The model under review builds one solid part; all positions refer to its coordinate system, in mm. A direction names the side the tool comes from. Give positions to 0.01 mm unless a question says otherwise; leave off trailing zeros. Order: outer loops, then holes, each group sorted by start corner. A loop starts at its lowest first (then second) coordinate and runs counter-clockwise, first axis right, second up. Notation, with made-up numbers: (48, 38) - (101, 38) arc R35 cw to (101, 72) - close; hole circle Ø10 at (35, -25.5). An arc over 180 degrees is marked (long way). Use CSV: the item, a comma, the result in double quotes. Start each with the question number.
```python
from build123d import *

# Parameters (mm, degrees)
F0_W     = 215.9
F0_H     = 50.8
F0_R     = 2.5527
F0_R_2   = 14.2875
F1_DEPTH = 25.4
F2_W     = 22.225
F2_H     = 47.625
F3_DEPTH = 215.901
F4_R     = 2.5527
F5_DEPTH = 50.801


with BuildPart() as f1:
    # F0 (on Front) → F1 (new body)
    with BuildSketch(Plane.XZ):
        Rectangle(F0_W, F0_H)
        with Locations((-57.15, -12.7)):
            Circle(F0_R, mode=Mode.SUBTRACT)
        with Locations((-31.75, -12.7)):
            Circle(F0_R, mode=Mode.SUBTRACT)
        with Locations((-6.35, -12.7)):
            Circle(F0_R, mode=Mode.SUBTRACT)
        with Locations((-82.55, 0)):
            Circle(F0_R_2, mode=Mode.SUBTRACT)
        with Locations((19.05, -12.7)):
            Circle(F0_R, mode=Mode.SUBTRACT)
        with Locations((44.45, -12.7)):
            Circle(F0_R, mode=Mode.SUBTRACT)
        with Locations((69.85, -12.7)):
            Circle(F0_R, mode=Mode.SUBTRACT)
        with Locations((95.25, -12.7)):
            Circle(F0_R, mode=Mode.SUBTRACT)
        with Locations((-57.15, 12.7)):
            Circle(F0_R, mode=Mode.SUBTRACT)
        with Locations((-31.75, 12.7)):
            Circle(F0_R, mode=Mode.SUBTRACT)
        with Locations((-6.35, 12.7)):
            Circle(F0_R, mode=Mode.SUBTRACT)
        with Locations((19.05, 12.7)):
            Circle(F0_R, mode=Mode.SUBTRACT)
        with Locations((44.45, 12.7)):
            Circle(F0_R, mode=Mode.SUBTRACT)
        with Locations((69.85, 12.7)):
            Circle(F0_R, mode=Mode.SUBTRACT)
        with Locations((95.25, 12.7)):
            Circle(F0_R, mode=Mode.SUBTRACT)
    extrude(amount=F1_DEPTH)

    # F2 (on face) → F3 (cut, through all)
    with BuildSketch(Plane(origin=(-107.95, 0, 0), x_dir=(0, -1, 0), z_dir=(-1, 0, 0))):
        with Locations((12.7, 0)):
            Rectangle(F2_W, F2_H)
    extrude(amount=-F3_DEPTH, mode=Mode.SUBTRACT)

    # F4 (on face) → F5 (cut, through all)
    with BuildSketch(Plane.XY.offset(25.4)):
        with Locations((-95.25, -12.7)):
            Circle(F4_R)
        with Locations((-57.15, -12.7)):
            Circle(F4_R)
        with Locations((-19.05, -12.7)):
            Circle(F4_R)
        with Locations((19.05, -12.7)):
            Circle(F4_R)
        with Locations((57.15, -12.7)):
            Circle(F4_R)
        with Locations((95.25, -12.7)):
            Circle(F4_R)
    extrude(amount=-F5_DEPTH, mode=Mode.SUBTRACT)


solid = f1.part
```
1. Consider section B-B (x = 44.45). Give the boundary of the cut face in (y, z).
2. Consider section A-A (z = -18). Give the boundary of the cut face in (x, y).
3. Clearance check with flat-ended pins moving along their axes: pin 1 (8 mm diameter, centred on x = -31.75, z = 12.7, fed in from -Y); pin 2 (4 mm diameter, centred on x = 69.85, z = -12.7, fed in from -Y). State where each tip first meets the part, or that it passes through.
4. Consider section D-D (z = 0). Give the boundary of the cut face in (x, y).
5. Mouldability with a two-part tool opening along Y and no side actions: class faces 3 (the face through (17.02, -14.25, -24.6)), 4 (the face through (-6.903, -24.595, 10.208)) as pulls with the +Y half, pulls with the -Y half, needs draft (parallel to the pull), parting line crosses it, or undercut.
6. Consider section C-C (y = -5.25). Give the boundary of the cut face in (x, z).
7. Tool access review of faces 1 (the face through (18.497, -24.595, 10.208)), 2 (the face through (-2, -23.812, 0)): name each direction out of +Z, -Z, +X, -X, +Y, -Y from which nothing blocks a thin tool from reaching the whole face with its end or side.
8. To check wall thickness, follow L1, parallel to Z at x = 95.25, y = -24.55; L2, parallel to Y at x = 95.25, z = -24.95; L3, parallel to Z at x = -12.5, y = -12.5. State the ranges of each line that lie inside material, in increasing order. Write a range as [from, to].
Answers follow:
1,outline,"(-25.4, -25.4) - (0, -25.4) - (0, -15.25) - (-1.59, -15.25) - (-1.59, -23.81) - (-23.81, -23.81) - (-23.81, -15.25) - (-25.4, -15.25) - close; (-25.4, -10.15) - (-23.81, -10.15) - (-23.81, 10.15) - (-25.4, 10.15) - close; (-25.4, 15.25) - (-23.81, 15.25) - (-23.81, 23.81) - (-1.59, 23.81) - (-1.59, 15.25) - (0, 15.25) - (0, 25.4) - (-25.4, 25.4) - close; (-1.59, -10.15) - (0, -10.15) - (0, 10.15) - (-1.59, 10.15) - close"
2,outline,"(-107.95, -25.4) - (107.95, -25.4) - (107.95, -23.81) - (-107.95, -23.81) - close; (-107.95, -1.59) - (107.95, -1.59) - (107.95, 0) - (-107.95, 0) - close"
3,pin 1,"stops at y = -25.4"
3,pin 2,"passes through"
4,outline,"(-107.95, -25.4) - (-96.84, -25.4) - (-96.84, -23.81) - (-107.95, -23.81) - close; (-107.95, -1.59) - (-96.84, -1.59) - (-96.84, 0) - (-107.95, 0) - close; (-68.26, -25.4) - (107.95, -25.4) - (107.95, -23.81) - (-68.26, -23.81) - close; (-68.26, -1.59) - (107.95, -1.59) - (107.95, 0) - (-68.26, 0) - close"
5,face 3,"undercut"
5,face 4,"needs draft"
6,outline,"(-107.95, -25.4) - (107.95, -25.4) - (107.95, -23.81) - (-107.95, -23.81) - close; (-107.95, 23.81) - (107.95, 23.81) - (107.95, 25.4) - (-107.95, 25.4) - close"
7,face 1,"+Y, -Y"
7,face 2,"+X, -X"
8,L1,"z = [-25.4, -15.25], [-10.15, 10.15], [15.25, 25.4]"
8,L2,"y = [-25.4, -15.25], [-10.15, 0]"
8,L3,"z = [-25.4, -23.81], [23.81, 25.4]"
